Build history of the part. All positions in model axes, mm. A direction names the side the tool comes from. Coordinates: 2 decimals unless noted, no trailing zeros. Write each loop counter-clockwise with the first axis right and the second up, starting at its lowest first coordinate (ties: lowest second). Pieces come first, ordered by that corner, then holes.
from build123d import *

# Parameters (mm, degrees)
BASE_SHAPE_BASE_DEPTH        = 20
BASE_SHAPE_EXTENSION_DEPTH   = 40
BASE_SHAPE_FINISH_SKETCH_W   = 10
BASE_SHAPE_FINISH_SKETCH_H   = 40
BASE_SHAPE_FINISH_DEPTH      = 40
ROD_HOLE_D8_Z_D              = 8
ROD_HOLE_D8_Z_DEPTH          = 40
ROD_HOLE_D8_Z_CSINK_D        = 8.2
ROD_HOLE_D8_Z_CSINK_ANGLE    = 60
ROD_HOLE_D8_Z_TIP            = 2.403442476
ROD_HOLE_D8_X_D              = 8
ROD_HOLE_D8_X_DEPTH          = 40
ROD_HOLE_D8_X_CSINK_D        = 8.2
ROD_HOLE_D8_X_CSINK_ANGLE    = 60
ROD_HOLE_D8_X_TIP            = 2.403442476
ROD_HOLE_D8_Y_D              = 8
ROD_HOLE_D8_Y_DEPTH          = 40
ROD_HOLE_D8_Y_CSINK_D        = 8.2
ROD_HOLE_D8_Y_CSINK_ANGLE    = 60
ROD_HOLE_D8_Y_TIP            = 2.403442476
OUTER_CHAMFERS_SIZE          = 5
INNER_SMALLER_CHAMFERS_SIZE  = 1
LARGE_CHAMFERS_SIZE          = 20
HULL_PART_HOLES_M3_START     = 10
HULL_PART_HOLES_M3_OUTLINE_R = 1.7
HULL_PART_HOLES_M3_DEPTH     = 10
HULL_PART_NUT_HOLE_DEPTH     = 5


# Read off the part's stored shape, not the designer's step: hull_part_holes_m3
with BuildPart() as part:
    # base_shape_sketch → base_shape_base (new body)
    with BuildSketch(Plane.XY):
        Polygon((0, 0), (60, 0), (60, 20), (20, 20), (20, 60), (0, 60), align=None)
    extrude(amount=BASE_SHAPE_BASE_DEPTH)

    # base_shape_extension_sketch → base_shape_extension (add)
    with BuildSketch(Plane.XY.offset(20)):
        Polygon((20, 60), (20, 20), (60, 20), (60, 10), (20, 10), (20, 0), (0, 0), (0, 20), (10, 20), (10, 60), align=None)
    extrude(amount=BASE_SHAPE_EXTENSION_DEPTH)

    # base_shape_finish_sketch → base_shape_finish (add)
    with BuildSketch(Plane(origin=(20, 0, 0), x_dir=(0, 0, -1), z_dir=(1, 0, 0))):
        with Locations((-15, 40)):
            Rectangle(BASE_SHAPE_FINISH_SKETCH_W, BASE_SHAPE_FINISH_SKETCH_H)
    extrude(amount=BASE_SHAPE_FINISH_DEPTH)

    # rod_hole_d8_z
    with Locations(Plane.XY.offset(60)):
        with Locations((10, 10)):
            CounterSinkHole(ROD_HOLE_D8_Z_D / 2, ROD_HOLE_D8_Z_CSINK_D / 2, depth=ROD_HOLE_D8_Z_DEPTH, counter_sink_angle=ROD_HOLE_D8_Z_CSINK_ANGLE)
            with Locations((0, 0, -(ROD_HOLE_D8_Z_DEPTH + ROD_HOLE_D8_Z_TIP / 2))):  # 118° drill point
                Cone(0, ROD_HOLE_D8_Z_D / 2, ROD_HOLE_D8_Z_TIP, mode=Mode.SUBTRACT)

    # rod_hole_d8_x
    with Locations(Plane(origin=(60, 0, 0), x_dir=(0, 0, -1), z_dir=(1, 0, 0))):
        with Locations((-10, 10)):
            CounterSinkHole(ROD_HOLE_D8_X_D / 2, ROD_HOLE_D8_X_CSINK_D / 2, depth=ROD_HOLE_D8_X_DEPTH, counter_sink_angle=ROD_HOLE_D8_X_CSINK_ANGLE)
            with Locations((0, 0, -(ROD_HOLE_D8_X_DEPTH + ROD_HOLE_D8_X_TIP / 2))):  # 118° drill point
                Cone(0, ROD_HOLE_D8_X_D / 2, ROD_HOLE_D8_X_TIP, mode=Mode.SUBTRACT)

    # rod_hole_d8_y
    with Locations(Plane(origin=(0, 60, 0), x_dir=(1, 0, 0), z_dir=(0, 1, 0))):
        with Locations((10, -10)):
            CounterSinkHole(ROD_HOLE_D8_Y_D / 2, ROD_HOLE_D8_Y_CSINK_D / 2, depth=ROD_HOLE_D8_Y_DEPTH, counter_sink_angle=ROD_HOLE_D8_Y_CSINK_ANGLE)
            with Locations((0, 0, -(ROD_HOLE_D8_Y_DEPTH + ROD_HOLE_D8_Y_TIP / 2))):  # 118° drill point
                Cone(0, ROD_HOLE_D8_Y_D / 2, ROD_HOLE_D8_Y_TIP, mode=Mode.SUBTRACT)

    # outer_chamfers
    outer_chamfers_edges = [part.edges().sort_by_distance(p)[0] for p in [
        (0, 0, 30),
        (30, 0, 0),
        (0, 30, 0),
    ]]
    chamfer(outer_chamfers_edges, length=OUTER_CHAMFERS_SIZE)

    # inner_smaller_chamfers
    inner_smaller_chamfers_edges = [part.edges().sort_by_distance(p)[0] for p in [
        (0, 60, 12.5),
        (60, 0, 12.5),
        (60, 5, 20),
        (40, 0, 20),
        (5, 60, 20),
        (0, 20, 40),
        (20, 0, 40),
        (5, 20, 60),
        (0, 12.5, 60),
        (20, 5, 60),
        (20, 60, 5),
        (0, 40, 20),
        (60, 20, 5),
        (12.5, 60, 0),
        (20, 40, 0),
        (40, 20, 0),
        (12.5, 0, 60),
        (2.5, 2.5, 60),
        (60, 12.5, 0),
        (60, 2.5, 2.5),
        (2.5, 60, 2.5),
    ]]
    chamfer(inner_smaller_chamfers_edges, length=INNER_SMALLER_CHAMFERS_SIZE)

    # large_chamfers
    large_chamfers_edges = [part.edges().sort_by_distance(p)[0] for p in [
        (15, 60, 60),
        (60, 15, 60),
        (60, 60, 15),
    ]]
    chamfer(large_chamfers_edges, length=LARGE_CHAMFERS_SIZE)

    # hull_part_holes_m3 outline → hull_part_holes_m3 (cut)
    with BuildSketch(Plane.YZ.offset(HULL_PART_HOLES_M3_START)):
        with Locations((45, 30)):
            Circle(HULL_PART_HOLES_M3_OUTLINE_R)
        with Locations((30, 45)):
            Circle(HULL_PART_HOLES_M3_OUTLINE_R)
    hull_part_holes_m3 = extrude(amount=HULL_PART_HOLES_M3_DEPTH, mode=Mode.SUBTRACT)

    # Sketch12 → hull_part_nut_hole (cut)
    with BuildSketch(Plane(origin=(20, 0, 0), x_dir=(0, 0, -1), z_dir=(1, 0, 0))):
        Polygon((-30, 48.175426481), (-32.75, 46.58771324), (-32.75, 43.41228676), (-30, 41.824573519), (-27.25, 43.41228676), (-27.25, 46.58771324), align=None)
        Polygon((-45, 33.175426481), (-47.75, 31.58771324), (-47.75, 28.41228676), (-45, 26.824573519), (-42.25, 28.41228676), (-42.25, 31.58771324), align=None)
    hull_part_nut_hole = extrude(amount=-HULL_PART_NUT_HOLE_DEPTH, mode=Mode.SUBTRACT)

    # hull_part_holes_mirror_x: hull_part_holes_m3, hull_part_nut_hole across plane
    add(hull_part_holes_m3.mirror(Plane(origin=(0, 0, 0), x_dir=(0.7071067811865482, 0, 0.7071067811865468), z_dir=(-0.707106781186547, 0, 0.7071067811865481))), mode=Mode.SUBTRACT)
    add(hull_part_nut_hole.mirror(Plane(origin=(0, 0, 0), x_dir=(0.7071067811865482, 0, 0.7071067811865468), z_dir=(-0.707106781186547, 0, 0.7071067811865481))), mode=Mode.SUBTRACT)

    # hull_part_holes_mirror_y: hull_part_holes_m3, hull_part_nut_hole across plane
    add(hull_part_holes_m3.mirror(Plane(origin=(0, 0, 0), x_dir=(0, 0, 1), z_dir=(-0.7071067811865482, 0.7071067811865469, 0))), mode=Mode.SUBTRACT)
    add(hull_part_nut_hole.mirror(Plane(origin=(0, 0, 0), x_dir=(0, 0, 1), z_dir=(-0.7071067811865482, 0.7071067811865469, 0))), mode=Mode.SUBTRACT)


solid = part.part
(1) Probe L1, parallel to Z at x = 11.45, y = 30; L2, parallel to Z at x = 45, y = 11; L3, parallel to X at y = 30, z = 13.4. List the from-to ranges inside material, lowest first.
(2) Flat gauge pins, fed straight in: P1, Ø4.5, axis at y = 30, z = 45, coming from the +X side; P2, Ø6, axis at x = 29, y = 44.5, coming from the +Z side; P3, Ø12, axis at y = 39, z = 44.5, coming from the +X side; P4, Ø3, axis at x = 30, z = 45, coming from the +Y side. Where does each tip first touch, or does it go through?
(3) Slice it at A-A, the plane y = 50. List the corners of the cut face in (x, z).
(4) Two-plate mould, pull along Y, no slides. Class faces 1 (the conical face through (10.373, 18.014, 9.414)), 2 (the flat face through (42.61, 17.54, 28.64)), 3 (the conical face through (18.014, 10.209, 9.337)): pulls with the +Y half, pulls with the -Y half, needs draft (parallel to the pull), parting line crosses it, or undercut.
(5) 3-axis set-ups, long thin cutter, end or side, ignore diameter. For faces 4 (the flat face through (17.535, 27.63, 46.394)), 5 (the flat face through (47.39, 17.54, 31.36)), 6 (the flat face through (5, 40, 20)), 7 (the flat face through (42.25, 30, 18)), 8 (the flat face through (20, 40, 40)): which of +Z, -Z, +X, -X, +Y, -Y reach the whole face in a straight line?
Results:
1. L1: z = 0 to 6.27, 13.73 to 43.3, 46.7 to 60
1. L2: z = 0 to 6.13, 13.87 to 28.3, 31.7 to 55
1. L3: x = 0 to 7.89, 12.11 to 43.3, 46.7 to 60
2. P1: stops at x = 15
2. P2: stops at z = 20
2. P3: stops at x = 20
2. P4: passes through
3. outline: (0, 5) - (5, 0) - (19, 0) - (20, 1) - (20, 10) - (50, 10) - (50, 20) - (20, 20) - (20, 50) - (10, 50) - (10, 20) - (1, 20) - (0, 19) - close; hole circle Ø8 at (10, 10)
4. face 1: pulls with the +Y half
4. face 2: needs draft
4. face 3: undercut
5. face 4: +X
5. face 5: +Y
5. face 6: +Z, -X, +Y
5. face 7: +Z
5. face 8: +Z, +X, +Y
